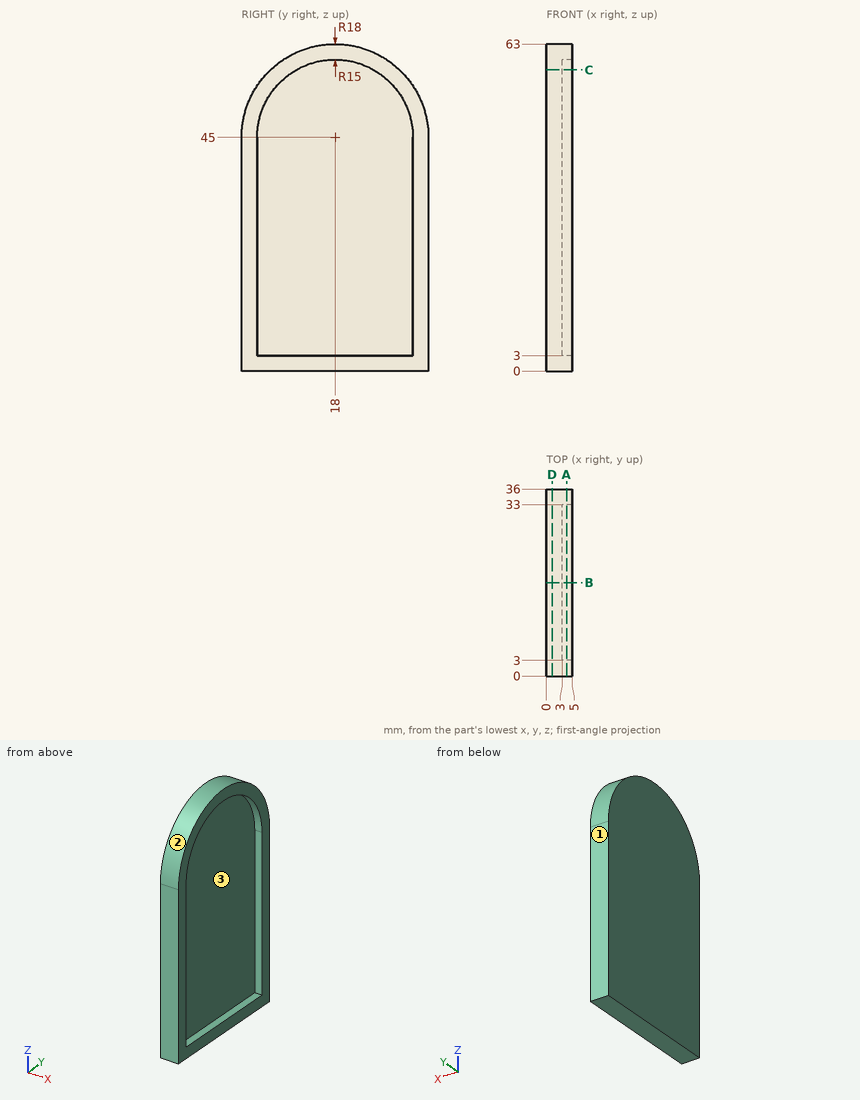
The drawing under review shows one solid part. Ordinate dimensions are in mm from its lowest x, y, z. Give positions to 0.01 mm unless a question says otherwise; leave off trailing zeros. Write each loop counter-clockwise with the first axis right and the second up, starting at its lowest first coordinate (ties: lowest second). Pieces come first, ordered by that corner, then holes. Notation, with made-up numbers: (-10.5, 41.5) -> (40.5, 41.5) arc R20 cw to (40.5, 69.5) -> close; hole circle Ø9 at (36.25, 12.25). An arc over 180 degrees is marked (long way). Use CSV: the item, a comma, the result in double quotes.
Q1. To check wall thickness, follow probe 1 along Y at (x, z) = (4.1, 16.5); probe 2 along X at (y, z) = (24.5, 29); probe 3 along Y at (x, z) = (4.45, 55). State the ranges of each line that lie inside material, in increasing order. Write a range as [from, to].
Conclusion:
probe 1,"[0, 3], [33, 36]"
probe 2,"[0, 3]"
probe 3,"[3.03, 6.82], [29.18, 32.97]"
Q2. Take a section at C-C, the plane z = 58. Write out the cut boundary in (x, y), then the cut area to 3 significant figures.
Conclusion:
outline,"(0, 5.55) -> (5, 5.55) -> (5, 10.52) -> (3, 10.52) -> (3, 25.48) -> (5, 25.48) -> (5, 30.45) -> (0, 30.45) -> close"
area,"94.6 mm2"
Q3. Take a section at D-D, the plane x = 1.1. Write out the cut boundary in (y, z).
Conclusion:
outline,"(0, 0) -> (36, 0) -> (36, 45) arc R18 ccw to (0, 45) -> close"
Q4. Take a section at B-B, the plane y = 18. Write out the cut boundary in (x, z).
Conclusion:
outline,"(0, 0) -> (5, 0) -> (5, 3) -> (3, 3) -> (3, 60) -> (5, 60) -> (5, 63) -> (0, 63) -> close"
Q5. For P1, Ø2, axis at x = 3.5, y = 25, coming from the +Z side; P2, Ø2, axis at x = 2.5, y = 12.5, coming from the +Z side; P3, Ø6, axis at y = 16.5, z = 38.5, coming from the +X side, all flat-tipped, find the tip position at first contact; note any pin that passes through.
Conclusion:
P1,"z = 61.97"
P2,"z = 62.43"
P3,"x = 3"
Q6. Take a section at A-A, the plane x = 3.9. Write out the cut boundary in (y, z), then the cut area to 3 significant figures.
Conclusion:
outline,"(0, 0) -> (36, 0) -> (36, 45) arc R18 ccw to (0, 45) -> close; hole (3, 3) -> (33, 3) -> (33, 45) arc R15 ccw to (3, 45) -> close"
area,"516 mm2"
Q7. Mouldability with a two-part tool opening along Y and no side actions: class the marked faces 1, 2 and 3 as pulls with the +Y half, pulls with the -Y half, needs draft (parallel to the pull), parting line crosses it, or undercut.
Conclusion:
face 1,"pulls with the +Y half"
face 2,"parting line crosses it"
face 3,"undercut"
